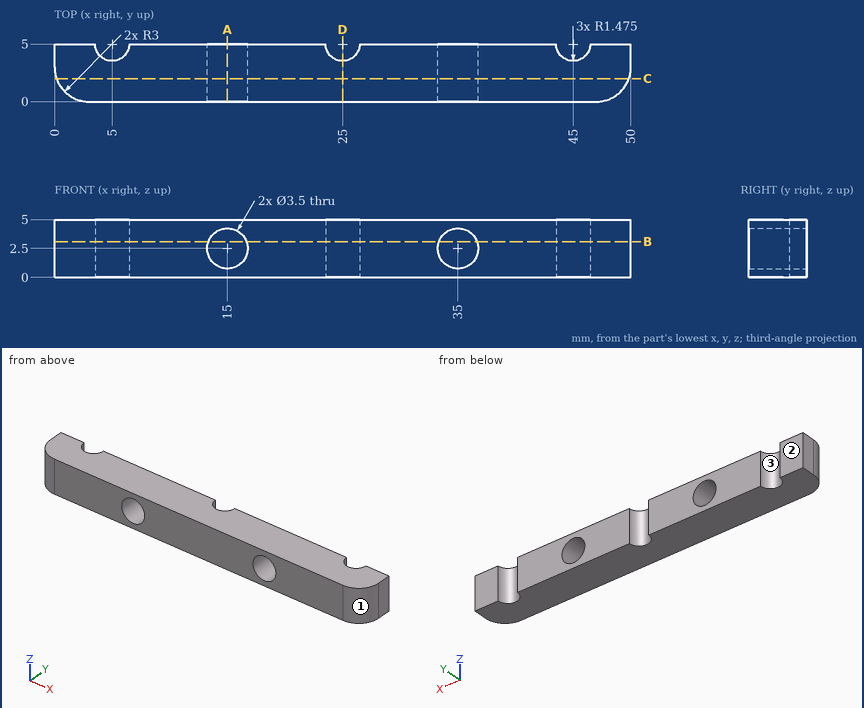
Print and shaded views of the part. All mm, measured from the part's lowest x, y and z. Round coordinates to 2 decimals unless told otherwise and drop trailing zeros. Write each loop counter-clockwise with the first axis right and the second up, starting at its lowest first coordinate (ties: lowest second). Pieces come first, ordered by that corner, then holes. Notation, with made-up numbers: M -12.5,-6.75 L 20.5,-6.75 A9 ccw 20.5,7.25 Z; hole C 30.25,55.25 d8. An arc over 180 degrees is marked long. Use a Markdown table: item, result. Add a question column.
1. Flat gauge pins, fed straight in: P1, Ø1.5, axis at y = 0.5, z = 3.5, coming from the -X side; P2, Ø1.5, axis at y = 1, z = 4, coming from the +X side. Where does each tip first touch, or does it go through?
2. Slice it at C-C on y = 2. Give the cut face in (x, z), then the cut area to 3 significant figures.
3. Drill centre lines: probe 1 along Z at (x, y) = (35, 3.8); probe 2 along X at (y, z) = (1.3, 3.85); probe 3 along X at (y, z) = (3.3, 3.05). Where is each one in solid material? Low to high.
4. Slice it at A-A on x = 15. Give the cut face in (y, z).
5. Slice it at D-D on x = 25. Give the cut face in (y, z) (3 decimals), then the cut area to 3 significant figures.
6. Pull direction X, two halves, no side cores. Call the marked faces 1, 2 and 3: released by +X, released by -X, zero draft, split by the parting line, or undercut.
7. Slice it at B-B on z = 3.1. Give the cut face in (x, y) (3 decimals).
Reply:
| question | item | result |
|---|---|---|
| 1 | P1 | stops at x = 0.56 |
| 1 | P2 | stops at x = 49.73 |
| 2 | outline | M 0.17,0 L 49.83,0 L 49.83,5 L 0.17,5 Z; hole C 15,2.5 d3.5; hole C 35,2.5 d3.5 |
| 2 | area | 229 mm^2 |
| 3 | probe 1 | z = 0 to 0.75, 4.25 to 5 |
| 3 | probe 2 | x = 0.53 to 13.89, 16.11 to 33.89, 36.11 to 49.47 |
| 3 | probe 3 | x = 0 to 13.34, 16.66 to 33.34, 36.66 to 50 |
| 4 | outline | M 0,0 L 5,0 L 5,0.75 L 0,0.75 Z; M 0,4.25 L 5,4.25 L 5,5 L 0,5 Z |
| 5 | outline | M 0,0 L 3.525,0 L 3.525,5 L 0,5 Z |
| 5 | area | 17.6 mm^2 |
| 6 | face 1 | released by +X |
| 6 | face 2 | zero draft |
| 6 | face 3 | undercut |
| 7 | outline | M 0,3 A3 ccw 3,0 L 13.356,0 L 13.356,5 L 6.475,5 A1.475 cw 3.525,5 L 0,5 Z; M 16.644,0 L 33.356,0 L 33.356,5 L 26.475,5 A1.475 cw 23.525,5 L 16.644,5 Z; M 36.644,0 L 47,0 A3 ccw 50,3 L 50,5 L 46.475,5 A1.475 cw 43.525,5 L 36.644,5 Z |
